Here's how the part is built. I have some questions about the finished solid (model axes, mm). A direction names the side the tool comes from. Round coordinates to 2 decimals unless told otherwise and drop trailing zeros. Order: outer loops, then holes, each group sorted by start corner. A loop starts at its lowest first (then second) coordinate and runs counter-clockwise, first axis right, second up. Notation, with made-up numbers: M 24,-34 L 77,-34 A22 ccw 77,-8 Z; hole C 63.25,19 d4. An arc over 180 degrees is marked long. Answer as CSV lines item,"result". Start each with the question number.
Autodesk Inventor part; units mm, degrees
ref_plane "YZ Plane" through (0, 0, 0) normal (1, 0, 0) x (0, 1, 0)
ref_plane "XZ Plane" through (0, 0, 0) normal (0, 1, 0) x (-1, 0, 0)
ref_plane "XY Plane" through (0, 0, 0) normal (0, 0, 1) x (1, 0, 0)
sketch "Sketch1" plane through (0, 0, 0) normal (0, 0, 1) x (1, 0, 0)
  line L0 (0, 0) -> (0, 3.9)
  line L1 (0, 3.9) -> (-17.7557, 3.9)
  line L2 (-17.7557, 3.9) -> (-2.7557, 3.9)
  line L3 (-17.7557, 3.9) -> (-17.7557, 13.9)
  line L4 (-17.7557, 13.9) -> (-19.7557, 13.9)
  line L5 (-19.7557, 13.9) -> (-19.7557, 3.9)
  line L6 (-19.7557, 3.9) -> (-34.7557, 3.9)
  line L7 (-34.7557, 3.9) -> (-64.7557, 3.9)
  line L8 (-64.7557, 3.9) -> (-64.7557, 0)
  line L9 (-64.7557, 0) -> (0, 0)
  dimension "d0" = 3.9
  dimension "d1" = 15
  dimension "d2" = 10
  dimension "d3" = 2
  dimension "d4" = 10
  dimension "d5" = 15
  dimension "d6" = 30
revolve "Revolution1" add sketch "Sketch1" angle 360 about axis through (-64.7557, 0, 0) along (1, 0, 0)
fillet "Fillet1" radius 0.2 2 edges at (-19.7557, -13.9, 0) (-17.7557, -13.9, 0)
properties part number "axlie"
Item 1: For P1, Ø8, axis at y = 3, z = 3, coming from the -X side; P2, Ø3, axis at x = -50, y = -1, coming from the -Z side; P3, Ø8, axis at x = -54.5, z = 10, coming from the +Y side; P4, Ø3, axis at y = 3, z = -7.5, coming from the -X side, each with a flat end and sliding along its axis, tell me the tip position at first contact or that it passes through.
Item 2: If I drill on line 1 along X through (y, z) = (2.5, -8.5); line 2 along Y through (x, z) = (-20, 1); line 3 along Z through (x, y) = (-18.5, -6.25), over which ranges is the centre line in solid material (lowest first)?
Item 3: If we section it at C-C on x = -40: Please give me the cut outline in (y, z), and give its area (3 significant figures).
Item 4: Which directions (+Z, -Z, +X, -X, +Y, -Y) give clear straight access to the entire face, cutting with the end or side of a thin tool? Please do faces 1 (the flat face through (0, 0, 0)), 2 (the cylindrical face through (-9, -2.87, -2.64)), 3 (the cylindrical face through (-42.57, -2.87, -2.64)).
Item 5: If we section it at A-A on z = 0: Please give me the cut outline in (x, y).
Geometry says:
1,P1,"x = -64.76"
1,P2,"z = -3.9"
1,P3,"through"
1,P4,"x = -19.76"
2,line 1,"-19.76 to -17.76"
2,line 2,"-3.77 to 3.77"
2,line 3,"-12.42 to 12.42"
3,outline,"C 0,0 d7.8"
3,area,"47.8 mm²"
4,face 1,"+Z, -Z, +X, +Y, -Y"
4,face 2,"+X"
4,face 3,"-X"
5,outline,"M -64.76,-3.9 L -19.76,-3.9 L -19.76,-13.7 A0.2 ccw -19.56,-13.9 L -17.96,-13.9 A0.2 ccw -17.76,-13.7 L -17.76,-3.9 L 0,-3.9 L 0,3.9 L -17.76,3.9 L -17.76,13.7 A0.2 ccw -17.96,13.9 L -19.56,13.9 A0.2 ccw -19.76,13.7 L -19.76,3.9 L -64.76,3.9 Z"
